Geometry: final body of the model. Coordinates: model frame, mm. A direction names the side the tool comes from. Round coordinates to 2 decimals unless told otherwise and drop trailing zeros. Order: outer loops, then holes, each group sorted by start corner. A loop starts at its lowest first (then second) coordinate and runs counter-clockwise, first axis right, second up. Notation, with made-up numbers: M 5,13.5 L 58,13.5 A15 ccw 58,34.5 Z; hole C -9.75,-15.5 d8. An arc over 180 degrees is marked long. Return JSON: item names as keys, results as strings. Group by question number.
Q1. Ray query, probe 1 along Z at (x, y) = (56.5, 2.1); probe 2 along X at (y, z) = (2.45, 0.5). Return the intervals inside material, ascending.
Q2. Access query for faces 1 (the face through (26, 2.7, -35)), 2 (the face through (26, 1.1, 1)), 3 (the face through (26, 2.7, 1)), 4 (the face through (51, 2, -35)), 5 (the face through (51, 2, 1)). Directions: +Z, -Z, +X, -X, +Y, -Y. A direction counts if a zero-diameter tool reaches every point of the face in a straight line with its end or side. Return the directions, or none.
Q3. Cut plane A-A on x = 41.5. Output: boundary loops of the cut face in (y, z), and give its area (3 significant figures).
Q4. Contact query for flat-ended pins moving along their axis: pin 1 (1.9 mm diameter, centred on x = 22, z = -35, fed in from +Y); pin 2 (1.5 mm diameter, centred on x = 49.5, y = 0.5, fed in from -Z); pin 3 (1.4 mm diameter, centred on x = 36, z = -35, fed in from -Y); pin 4 (0.8 mm diameter, centred on y = 2, z = 0.5, fed in from +X). Output: stop coordinate, or through.
```python
from build123d import *

# Parameters (mm, degrees)
SKETCH_1_W      = 65
SKETCH_1_H      = 34
EXTRUDE_1_DEPTH = 3.8
SKETCH_2_W      = 51
SKETCH_2_H      = 1.6
EXTRUDE_2_DEPTH = 1.7


with BuildPart() as part:
    # 草图1 → 凸台-拉伸1 (new body)
    with BuildSketch(Plane(origin=(0, 0, 0), x_dir=(1, 0, 0), z_dir=(0, 1, 0))):
        with Locations((32.5, 17)):
            Rectangle(SKETCH_1_W, SKETCH_1_H)
    extrude(amount=EXTRUDE_1_DEPTH)

    # 草图2 → 凸台-拉伸2 (add)
    with BuildSketch(Plane(origin=(0, 0, -34), x_dir=(-1, 0, 0), z_dir=(0, 0, -1))):
        with Locations((-25.5, 1.9)):
            Rectangle(SKETCH_2_W, SKETCH_2_H)
    extrude_2 = extrude(amount=EXTRUDE_2_DEPTH)

    # 镜向1: 凸台-拉伸2 across plane
    add(extrude_2.mirror(Plane.XY.offset(-17)))


solid = part.part
```
Result sheet:
{
 "1": {"probe 1": "z = -34 to 0", "probe 2": "x = 0 to 51"},
 "2": {"face 1": "-Z, +X, -X, +Y", "face 2": "+Z, +X, -X, -Y", "face 3": "+Z, +X, -X, +Y", "face 4": "-Z, +X, +Y, -Y", "face 5": "+Z, +X, +Y, -Y"},
 "3": {"outline": "M 0,-34 L 1.1,-34 L 1.1,-35.7 L 2.7,-35.7 L 2.7,-34 L 3.8,-34 L 3.8,0 L 2.7,0 L 2.7,1.7 L 1.1,1.7 L 1.1,0 L 0,0 Z", "area": "135 mm²"},
 "4": {"pin 1": "stops at y = 2.7", "pin 2": "stops at z = -35.7", "pin 3": "stops at y = 1.1", "pin 4": "stops at x = 51"}
}
